Autodesk Inventor part; units mm, degrees
ref_plane "YZ Plane" through (0, 0, 0) normal (1, 0, 0) x (0, 1, 0)
ref_plane "XZ Plane" through (0, 0, 0) normal (0, 1, 0) x (-1, 0, 0)
ref_plane "XY Plane" through (0, 0, 0) normal (0, 0, 1) x (1, 0, 0)
sketch "Sketch9" plane through (0, 0, 0) normal (0, 1, 0) x (-1, 0, 0)
  line L0 (0, 0) -> (900, 0)
  line L1 (900, 0) -> (900, -2000)
  line L2 (900, -2000) -> (0, -2000)
  line L3 (0, -2000) -> (0, 0)
  line L4 (900, -2000) -> (800, -2000)
  line L5 (800, -2000) -> (800, 3000)
  line L6 (800, 3000) -> (900, 3000)
  line L7 (900, 3000) -> (900, -2000)
  line L8 (0, -2000) -> (100, -2000)
  line L9 (100, -2000) -> (100, 0)
  line L10 (100, 0) -> (0, 0)
  line L11 (0, 0) -> (0, -2000)
  point P0 (100, -2000)
  point P1 (800, 0)
  dimension "d70" = 900
  dimension "d71" = 100
  dimension "d72" = 100
  dimension "d106" = 2000
extrude "Extrusion6" add sketch "Sketch9" along normal blind 1790 contours L0 L9 L2 L3 | L0 L1 L2 L5
sketch "Sketch10" plane through (0, 0, 0) normal (1, 0, 0) x (0, 0, -1)
  line L0 (0, 0) -> (0, 1790)
  line L1 (0, 1790) -> (5000, 1790)
  line L2 (5000, 1790) -> (5000, 1290)
  line L3 (5000, 1290) -> (0, 1290)
  line L4 (0, 1290) -> (0, 1790)
  line L5 (0, 1790) -> (5000, 1790)
  line L6 (5000, 1790) -> (5000, 1390)
  line L7 (5000, 1390) -> (0, 1390)
  line L8 (0, 1390) -> (0, 1790)
  line L9 (0, 1790) -> (5000, 1790)
  line L10 (5000, 1790) -> (5000, 1490)
  line L11 (5000, 1490) -> (0, 1490)
  line L12 (0, 1490) -> (0, 1790)
  line L13 (2000, 0) -> (0, 0)
  line L14 (0, 0) -> (500, 0)
  line L15 (500, 0) -> (500, 600)
  line L16 (500, 600) -> (0, 600)
  line L17 (0, 600) -> (0, 0)
  line L18 (2000, 0) -> (1500, 0)
  line L19 (1500, 0) -> (1500, 600)
  line L20 (1500, 600) -> (2000, 600)
  line L21 (2000, 600) -> (2000, 0)
  point P0 (5000, 1490)
  point P1 (0, 1490)
  point P2 (0, 1390)
  dimension "d83" = 500
  dimension "d84" = 500
  dimension "d85" = 600
  dimension "d86" = 600
extrude "Extrusion7" add sketch "Sketch10" against normal blind 900 contours L0 L11 L2 L7
sketch "Sketch13" plane through (0, 1790, 0) normal (0, 1, 0) x (1, 0, 0)
  line L0 (-900, 2000) -> (-900, 0)
  line L1 (0, 0) -> (0, 2000)
  line L2 (-900, 0) -> (0, 0)
  line L3 (0, 0) -> (0, 2000)
  line L4 (0, 2000) -> (-900, 2000)
  line L5 (-900, 2000) -> (-900, 0)
  point P0 (0, 4500)
extrude "Extrusion9" cut sketch "Sketch13" against normal blind 290
sketch "Boceto15" plane through (0, 1490, -2000) normal (0, 1, 0) x (1, 0, 0)
  line L0 (-900, 0) -> (-900, 3000)
  line L1 (0, 0) -> (-100, 0)
  line L2 (-900, 3000) -> (0, 3000)
  line L3 (0, 3000) -> (0, 0)
  line L4 (0, 0) -> (-900, 0)
  line L5 (-900, 0) -> (-900, 3000)
  point P0 (0, -2000)
  point P1 (-900, 0)
  point P2 (-100, 0)
extrude "Extrusión11" cut sketch "Boceto15" against normal blind 1500
sketch "Boceto16" plane through (0, 0, 0) normal (1, 0, 0) x (0, 0, -1)
  line L0 (0, 0) -> (500, 0)
  line L1 (2000, 0) -> (0, 0)
  line L2 (2000, 0) -> (1500, 0)
  line L3 (0, 1390) -> (2000, 1390)
  line L4 (500, 0) -> (400, 0)
  line L5 (400, 0) -> (400, 1390)
  line L6 (400, 1390) -> (500, 1390)
  line L7 (500, 1390) -> (500, 0)
  line L8 (0, 0) -> (100, 0)
  line L9 (100, 0) -> (100, 1390)
  line L10 (100, 1390) -> (0, 1390)
  line L11 (0, 1390) -> (0, 0)
  line L12 (2000, 0) -> (1900, 0)
  line L13 (1900, 0) -> (1900, 1390)
  line L14 (1900, 1390) -> (2000, 1390)
  line L15 (2000, 1390) -> (2000, 0)
  line L16 (1500, 0) -> (1600, 0)
  line L17 (1600, 0) -> (1600, 1390)
  line L18 (1600, 1390) -> (1500, 1390)
  line L19 (1500, 1390) -> (1500, 0)
  point P0 (1600, 1390)
  point P1 (1900, 1390)
  point P2 (1500, 1390)
  dimension "d110" = 500
  dimension "d111" = 500
  dimension "d112" = 100
  dimension "d113" = 100
  dimension "d114" = 100
  dimension "d115" = 100
extrude "Extrusión12" cut sketch "Boceto16" against normal blind 1500 contours L9 L3 L5 L0 | L7 L3 L19 L1 | L17 L3 L13 L1
properties part number "B_Transportadora_Recta_5m" material "Aluminum 6061"
Design review of the part built by this model. Coordinates are the model's own, in mm. A direction names the side the tool comes from. Round coordinates to 2 decimals unless told otherwise and drop trailing zeros. Loops run counter-clockwise (first coordinate to the right, second up) from the corner with the lowest first, then second, coordinate; pieces in that order, holes last. Notation, with made-up numbers: (79.5, 74.5) -> (102.5, 74.5) arc R12 cw to (102.5, 90.5) -> close; hole circle Ø4 at (-38, 13). An arc over 180 degrees is marked (long way). Use one line per item in the form item = value. Start each with the question number.
Q1. We need section B-B on z = -1847. Give the boundary of the cut face in (x, y).
Q2. We need section C-C on x = -159. Give the boundary of the cut face in (y, z).
Q3. Machinability: for faces 1 (the face through (-445, 1490, -1014)), 2 (the face through (-849, 685, -400)), 3 (the face through (-800, 685, -451)), which of the approach directions +Z, -Z, +X, -X, +Y, -Y give a long, thin tool a straight path to every point of the face, cutting with its end or side? Answer none if there is none.
Q4. We need section A-A on y = 1368.5. State how many separate pieces and enclosed holes the cut face has, then the cut area to 3 significant figures.
Q5. Wall thickness on line 1 along Z through (x, y) = (-96, 1091); line 2 along X through (y, z) = (173, -1545); line 3 along Y through (x, z) = (-71, -114): over which ranges is each line inside the solid? List them lowest first. Write a range as [from, to].
Q6. For pin 1 Ø3 at (x, z) = (-610.5, -1708.5) entering from -Y; pin 2 Ø4 at (x, z) = (-530.5, -1085.5) entering from +Y, all flat-tipped, find the tip position at first contact; note any pin that passes through.
Calculated:
q1.outline = (-900, 1390) -> (0, 1390) -> (0, 1500) -> (-100, 1500) -> (-100, 1490) -> (-800, 1490) -> (-800, 1500) -> (-900, 1500) -> close
q2.outline = (1390, -2000) -> (1490, -2000) -> (1490, 0) -> (1390, 0) -> close
q3.face_1 = +Z, -Z, +Y
q3.face_2 = +X, -X, -Y
q3.face_3 = +Z, -Z, -Y
q4.separate_pieces = 8
q4.enclosed_holes = 0
q4.area = 80,000 mm²
q5.line_1 = [-2000, -1900], [-1600, -1500], [-500, -400], [-100, 0]
q5.line_2 = [-900, -800], [-100, 0]
q5.line_3 = [1390, 1500]
q6.pin_1 = 1390
q6.pin_2 = 1490
